Geometry check sheet. Reference: the model listing, model coordinates, mm. Face numbers are marked on the shaded views. Coordinates: 2 decimals unless noted, no trailing zeros. Order: outer loops, then holes, each group sorted by start corner. A loop starts at its lowest first (then second) coordinate and runs counter-clockwise, first axis right, second up. Notation, with made-up numbers: (-3, 59) - (42, 59) arc R9 ccw to (42, 64) - close; hole circle Ø11 at (4, 2). An arc over 180 degrees is marked (long way). Put each result on its own line as item: value.
from build123d import *

# Parameters (mm, degrees)
F1_DEPTH = 25.4


with BuildPart() as f1:
    # F0 (on Top) → F1 (new body)
    with BuildSketch(Plane.XY):
        with BuildLine():
            Line((0, 1.709418), (0, 0))
            Line((0, 0), (2.536132, 0))
            Line((2.536132, 0), (2.536132, 1.70942))
            Line((2.536132, 1.70942), (51.430943, 1.70942))
            Line((51.430943, 1.70942), (51.430943, 0))
            Line((51.430943, 0), (53.967075, 0))
            Line((53.967075, 0), (53.967075, 1.709418))
            ThreePointArc((53.967075, 1.709418), (52.363333, 3.541403), (51.430943, 5.790582))
            Line((51.430943, 5.790582), (2.536132, 5.790582))
            ThreePointArc((2.536132, 5.790582), (1.603742, 3.541403), (0, 1.709418))
        make_face()
    extrude(amount=F1_DEPTH)


solid = f1.part
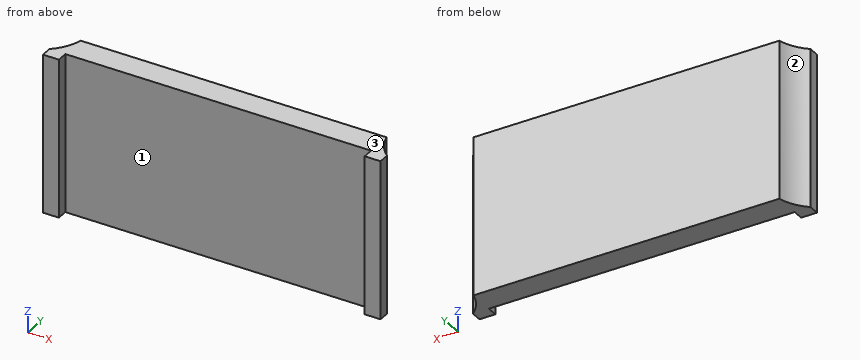
Q1. Thickness scan on L1, parallel to X at y = 1.35, z = 14; L2, parallel to Y at x = 22, z = 23; L3, parallel to X at y = 3.25, z = 22. Record the ranges inside material, lowest first. Write a range as [from, to].
Answer block:
L1: x = [0, 2.54], [51.43, 53.97]
L2: y = [1.71, 5.79]
L3: x = [1.41, 52.55]
Q2. Section check C-C on x = 4. Record the boundary of the cut face in (y, z).
Answer block:
outline: (1.71, 0) - (5.79, 0) - (5.79, 25.4) - (1.71, 25.4) - close
Q3. Section check A-A on y = 0.95. Record the boundary of the cut face in (x, z).
Answer block:
outline: (0, 0) - (2.54, 0) - (2.54, 25.4) - (0, 25.4) - close; (51.43, 0) - (53.97, 0) - (53.97, 25.4) - (51.43, 25.4) - close
Q4. Depth check by flat-ended pin: pin 1 Ø1.5 at (y, z) = (4.5, 9.5) entering from -X; pin 2 Ø12.5 at (x, z) = (24, 13) entering from -Y; pin 3 Ø1 at (y, z) = (2.5, 5) entering from -X. Enter the tip coordinate at first touch or a pass-through.
Answer block:
pin 1: stops at x = 1.73
pin 2: stops at y = 1.71
pin 3: stops at x = 0.33
Q5. Section check D-D on y = 4.1. Record the boundary of the cut face in (x, z), then the cut area to 3 significant figures.
Answer block:
outline: (1.92, 0) - (52.05, 0) - (52.05, 25.4) - (1.92, 25.4) - close
area: 1,270 mm^2
Q6. Section check B-B on z = 18.25. Record the boundary of the cut face in (x, y).
Answer block:
outline: (0, 0) - (2.54, 0) - (2.54, 1.71) - (51.43, 1.71) - (51.43, 0) - (53.97, 0) - (53.97, 1.71) arc R7.5 cw to (51.43, 5.79) - (2.54, 5.79) arc R7.5 cw to (0, 1.71) - close
Q7. Draft check along X on the marked faces 1, 2 and 3. Enter one of: pulls with the +X half, pulls with the -X half, needs draft (parallel to the pull), parting line crosses it, or undercut.
Answer block:
face 1: undercut
face 2: pulls with the -X half
face 3: needs draft
